from build123d import *

# Parameters (mm, degrees)
SKETCH1_W           = 14
SKETCH1_H           = 9.8
BOSS_EXTRUDE1_DEPTH = 3.3
SKETCH2_W           = 14
SKETCH2_H           = 9.8
SKETCH2_W_2         = 2.5
SKETCH2_H_2         = 3
SKETCH2_W_3         = 1
SKETCH2_H_3         = 1.5
CUT_EXTRUDE1_DEPTH  = 1.5
SKETCH3_W           = 14
SKETCH3_H           = 9.8
SKETCH3_W_2         = 1
SKETCH3_H_2         = 2
CUT_EXTRUDE2_DEPTH  = 1
SKETCH4_R           = 0.5
CUT_EXTRUDE3_DEPTH  = 1


with BuildPart() as part:
    # Sketch1 → Boss-Extrude1 (new body)
    with BuildSketch(Plane(origin=(0, 0, 0), x_dir=(1, 0, 0), z_dir=(0, 1, 0))):
        Rectangle(SKETCH1_W, SKETCH1_H)
    extrude(amount=BOSS_EXTRUDE1_DEPTH)

    # Sketch2 → Cut-Extrude1 (cut)
    with BuildSketch(Plane(origin=(0, 3.3, 0), x_dir=(1, 0, 0), z_dir=(0, 1, 0))):
        Rectangle(SKETCH2_W, SKETCH2_H)
        with Locations((-3.75, 2.9)):
            Rectangle(SKETCH2_W_2, SKETCH2_H_2, mode=Mode.SUBTRACT)
        with Locations((3.75, 2.9)):
            Rectangle(SKETCH2_W_2, SKETCH2_H_2, mode=Mode.SUBTRACT)
        with Locations((-1.5, -0.35)):
            Rectangle(SKETCH2_W_3, SKETCH2_H_3, mode=Mode.SUBTRACT)
    extrude(amount=-CUT_EXTRUDE1_DEPTH, mode=Mode.SUBTRACT)

    # Sketch3 → Cut-Extrude2 (cut)
    with BuildSketch(Plane.XZ):
        Rectangle(SKETCH3_W, SKETCH3_H)
        with Locations((-6, -1.4)):
            Rectangle(SKETCH3_W_2, SKETCH3_H_2, mode=Mode.SUBTRACT)
    extrude(amount=-CUT_EXTRUDE2_DEPTH, mode=Mode.SUBTRACT)

    # Sketch4 → Cut-Extrude3 (cut)
    with BuildSketch(Plane.XZ.offset(-1)):
        with Locations(Location((-5, 3.9, 0), (0, 0, 270))):
            Circle(SKETCH4_R)
        with Locations(Location((-2.5, 3.9, 0), (0, 0, 270))):
            Circle(SKETCH4_R)
        with Locations(Location((0, 3.9, 0), (0, 0, 270))):
            Circle(SKETCH4_R)
        with Locations(Location((2.5, 3.9, 0), (0, 0, 270))):
            Circle(SKETCH4_R)
        with Locations(Location((5, 3.9, 0), (0, 0, 270))):
            Circle(SKETCH4_R)
    extrude(amount=-CUT_EXTRUDE3_DEPTH, mode=Mode.SUBTRACT)


solid = part.part
Geometry check sheet. Reference: the model listing, model coordinates, mm. A direction names the side the tool comes from. Round coordinates to 2 decimals unless told otherwise and drop trailing zeros. Order: outer loops, then holes, each group sorted by start corner. A loop starts at its lowest first (then second) coordinate and runs counter-clockwise, first axis right, second up. Notation, with made-up numbers: (37.5, 77) -> (87.5, 77) arc R22 cw to (87.5, 99) -> close; hole circle Ø5 at (-14, -35). An arc over 180 degrees is marked (long way). Use one line per item in the form item = value.
1. Cross-section at C-C, the plane x = 0. Enter the section's corners in (y, z).
Working result:
outline = (1, -4.9) -> (1.8, -4.9) -> (1.8, 3.4) -> (1, 3.4) -> close; (1, 4.4) -> (1.8, 4.4) -> (1.8, 4.9) -> (1, 4.9) -> close
2. Set-up check for faces 5 (the face through (-5, 3, -3)), 6 (the face through (-4, 3, -4.4)), 7 (the face through (5, 3, -3)), 8 (the face through (4, 3, -1.4)): record each of +Z, -Z, +X, -X, +Y, -Y from which the full face is reachable in a straight line by a thin tool's end or side.
Working result:
face_5 = +Z, -Z, -X, +Y
face_6 = -Z, +X, -X, +Y
face_7 = +Z, -Z, +X, +Y
face_8 = +Z, +X, -X, +Y
3. Scan lines: line 1 along X through (y, z) = (1.3, 3.9); line 2 along Z through (x, y) = (-4, 1.95); line 3 along Y through (x, z) = (0.5, 4.25). Record each from-to range of solid material in increasing order. Write a range as from..to.
Working result:
line_1 = -7..-5.5, -4.5..-3, -2..-0.5, 0.5..2, 3..4.5, 5.5..7
line_2 = -4.4..-1.4
line_3 = 1..1.8
4. Go/stop test with flat-tipped pins: pin 1 (1.2 mm diameter, centred on y = 2.5, z = -2.5, fed in from -X); pin 2 (0.8 mm diameter, centred on x = -4, y = 2.5, fed in from -Z); pin 3 (0.8 mm diameter, centred on x = -6, y = 0.5, fed in from +Z). Record where each tip stops, or that it passes through.
Working result:
pin_1 = -5
pin_2 = -4.4
pin_3 = -0.4
5. Cross-section at D-D, the plane z = -3.5. Enter the section's corners in (x, y), plus the area to 3 significant figures.
Working result:
outline = (-7, 1) -> (7, 1) -> (7, 1.8) -> (5, 1.8) -> (5, 3.3) -> (2.5, 3.3) -> (2.5, 1.8) -> (-2.5, 1.8) -> (-2.5, 3.3) -> (-5, 3.3) -> (-5, 1.8) -> (-7, 1.8) -> close
area = 18.7 mm^2
6. Cross-section at B-B, the plane z = 3.9. Enter the section's corners in (x, y).
Working result:
outline = (-7, 1) -> (-5.5, 1) -> (-5.5, 1.8) -> (-7, 1.8) -> close; (-4.5, 1) -> (-3, 1) -> (-3, 1.8) -> (-4.5, 1.8) -> close; (-2, 1) -> (-0.5, 1) -> (-0.5, 1.8) -> (-2, 1.8) -> close; (0.5, 1) -> (2, 1) -> (2, 1.8) -> (0.5, 1.8) -> close; (3, 1) -> (4.5, 1) -> (4.5, 1.8) -> (3, 1.8) -> close; (5.5, 1) -> (7, 1) -> (7, 1.8) -> (5.5, 1.8) -> close
7. Cross-section at A-A, the plane y = 2.65. Enter the section's corners in (x, z).
Working result:
outline = (-5, -4.4) -> (-2.5, -4.4) -> (-2.5, -1.4) -> (-5, -1.4) -> close; (-2, -0.4) -> (-1, -0.4) -> (-1, 1.1) -> (-2, 1.1) -> close; (2.5, -4.4) -> (5, -4.4) -> (5, -1.4) -> (2.5, -1.4) -> close
8. Mould release check, pull along X, two halves, no side actions. Record for faces 1 (the face through (-6.5, 0.5, -1.4)), 2 (the face through (-0.192, 1.394, 3.438)), 3 (the face through (-1.5, 2.6, -0.4)), 4 (the face through (-4.85, 1.394, 3.423)): pulls with the +X half, pulls with the -X half, needs draft (parallel to the pull), parting line crosses it, or undercut.
Working result:
face_1 = pulls with the -X half
face_2 = undercut
face_3 = needs draft
face_4 = undercut
